For this review, take the finished solid that the model builds, in its own axes (mm). Coordinates: 2 decimals unless noted, no trailing zeros. Write each loop counter-clockwise with the first axis right and the second up, starting at its lowest first coordinate (ties: lowest second). Pieces come first, ordered by that corner, then holes. Notation, with made-up numbers: M -16,12.25 L 17,12.25 A20 ccw 17,48.25 Z; hole C 73,77.5 d7. An arc over 180 degrees is marked long. One line per question, with ' | ' between items.
from build123d import *

# Parameters (mm, degrees)
F0_W     = 70.1
F0_H     = 58
F1_DEPTH = 30
F2_R     = 10.025
F3_DEPTH = 30
F5_D     = 7.8


with BuildPart() as f1:
    # F0 (on Top) → F1 (new body)
    with BuildSketch(Plane.XY):
        with Locations((35.05, -29)):
            Rectangle(F0_W, F0_H)
    extrude(amount=F1_DEPTH)

    # F2 (on face) → F3 (cut)
    with BuildSketch(Plane.XY):
        with Locations((35.05, -33.0747030675)):
            Circle(F2_R)
    extrude(amount=F3_DEPTH, mode=Mode.SUBTRACT)

    # F5 (through all)
    with Locations(Plane.XZ.offset(58)):
        with Locations((35.05, 15)):
            Hole(F5_D / 2)


solid = f1.part
1. Clearance check with a flat-ended pin moving along its axis: P1, Ø3, axis at y = -31.5, z = 7.5, coming from the -X side. State where the tip first meets the part, or that it passes through.
Computed values:
P1: stops at x = 0
2. Take a section at A-A on x = 35.05. State the section outline as (y, z) points.
Computed values:
outline: M -58,0 L -43.1,0 L -43.1,11.1 L -58,11.1 Z; M -58,18.9 L -43.1,18.9 L -43.1,30 L -58,30 Z; M -23.05,0 L 0,0 L 0,11.1 L -23.05,11.1 Z; M -23.05,18.9 L 0,18.9 L 0,30 L -23.05,30 Z
3. Take a section at B-B on y = -40. State the section outline as (x, z) points.
Computed values:
outline: M 0,0 L 27.8,0 L 27.8,30 L 0,30 Z; M 42.3,0 L 70.1,0 L 70.1,30 L 42.3,30 Z
4. For line 1 along X through (y, z) = (-33, 2); line 2 along X through (y, z) = (-49, 15); line 3 along Z through (x, y) = (35.05, -7), list the stretches that pass through material, from the lowest coordinate up.
Computed values:
line 1: x = 0 to 25.03, 45.07 to 70.1 | line 2: x = 0 to 31.15, 38.95 to 70.1 | line 3: z = 0 to 11.1, 18.9 to 30
5. Draft analysis for pull direction Z (two halves, no side actions). For faces 1 (the cylindrical face through (31.33, -11.75, 16.17)), 2 (the flat face through (35, 0, 8)), 3 (the flat face through (35, -22, 30)), state which applies: pulls with the +Z half, pulls with the -Z half, needs draft (parallel to the pull), parting line crosses it, or undercut.
Computed values:
face 1: undercut | face 2: needs draft | face 3: pulls with the +Z half
6. Take a section at D-D on z = 10. State the section outline as (x, y) points (3 decimals), plus the area to 3 significant figures.
Computed values:
outline: M 0,-58 L 70.1,-58 L 70.1,0 L 0,0 Z; hole C 35.05,-33.075 d20.05 | area: 3,750 mm2
7. Take a section at C-C on y = -21. State the section outline as (x, z) points.
Computed values:
outline: M 0,0 L 70.1,0 L 70.1,30 L 0,30 Z; hole C 35.05,15 d7.8
